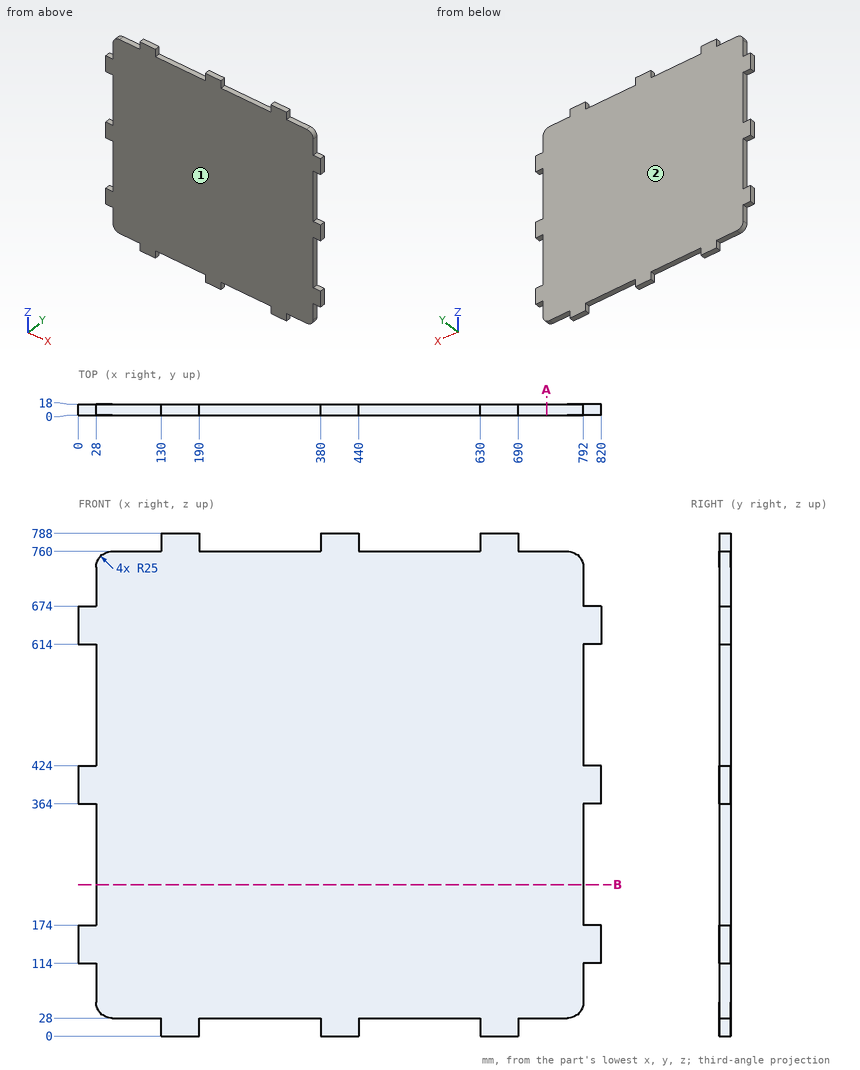
Print and shaded views of the part. All mm, measured from the part's lowest x, y and z. Coordinates: 2 decimals unless noted, no trailing zeros. Write each loop counter-clockwise with the first axis right and the second up, starting at its lowest first coordinate (ties: lowest second). Pieces come first, ordered by that corner, then holes.
(1) Flat gauge pins, fed straight in: pin 1 (5.5 mm diameter, centred on x = 802.5, y = 11, fed in from +Z); pin 2 (5 mm diameter, centred on y = 3.5, z = 518.5, fed in from +X); pin 3 (4 mm diameter, centred on x = 83.5, y = 13, fed in from +Z). Where does each tip first touch, or does it go through?
(2) Two-plate mould, pull along Y, no slides. Class the marked faces 1 and 2: +Y half, -Y half, draft (parallel to the pull), parting line (faces both ways), or undercut.
(3) Cut at B-B, the plane z = 237.5. List the corners of the cut face in (x, y), and give its area (3 significant figures).
(4) Drill centre lines: probe 1 along X at (y, z) = (13.5, 86); probe 2 along Z at (x, y) = (338.5, 13.5); probe 3 along Z at (x, y) = (50, 3.25). Where is each one in solid material? Low to high.
(5) Cut at A-A, the plane x = 734.5. List the corners of the cut face in (y, z), and give its area (3 significant figures).
Geometry says:
1. pin 1: stops at z = 674
1. pin 2: stops at x = 792
1. pin 3: stops at z = 760
2. face 1: -Y half
2. face 2: +Y half
3. outline: (28, 0) - (792, 0) - (792, 18) - (28, 18) - close
3. area: 13,800 mm2
4. probe 1: x = 28 to 792
4. probe 2: z = 28 to 760
4. probe 3: z = 28.18 to 759.82
5. outline: (0, 28) - (18, 28) - (18, 760) - (0, 760) - close
5. area: 13,200 mm2
